For this review, take the finished solid that the model builds, in its own axes (mm). Face numbers are marked on the shaded views. A direction names the side the tool comes from. Round coordinates to 2 decimals unless told otherwise and drop trailing zeros. Write each loop counter-clockwise with the first axis right and the second up, starting at its lowest first coordinate (ties: lowest second). Pieces come first, ordered by that corner, then holes. Notation, with made-up numbers: (-22, 55.5) -> (26, 55.5) arc R14 cw to (26, 66.5) -> close; hole circle Ø4 at (38, 22). An arc over 180 degrees is marked (long way). Answer in a Markdown table with one row per item.
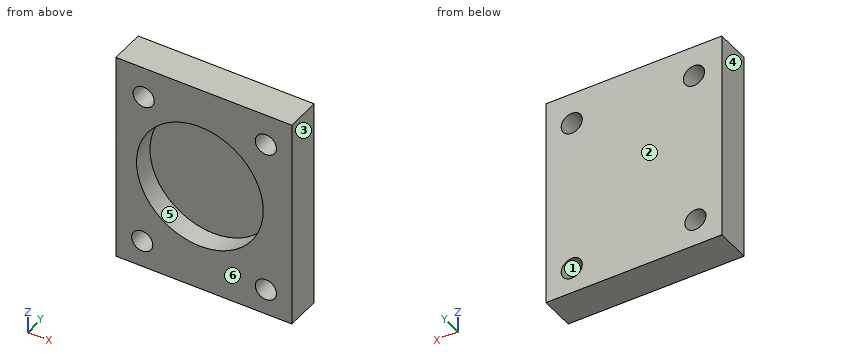
from build123d import *

# Parameters (mm, degrees)
F0_W     = 25
F0_H     = 30
F1_DEPTH = 5
F2_R     = 1.5
F3_DEPTH = 25
F4_R     = 9
F5_DEPTH = 3


with BuildPart() as f1:
    # F0 (on Front) → F1 (new body)
    with BuildSketch(Plane.XZ):
        with Locations((0.55913, 2.599103)):
            Rectangle(F0_W, F0_H)
    extrude(amount=F1_DEPTH)

    # F2 (on face) → F3 (cut)
    with BuildSketch(Plane.XZ.offset(5)):
        with Locations((-7.987171, 13.230707)):
            Circle(F2_R)
        with Locations((9.378917, 13.162337)):
            Circle(F2_R)
        with Locations((-8.192283, -8.579459)):
            Circle(F2_R)
        with Locations((9.378917, -8.716201)):
            Circle(F2_R)
    extrude(amount=-F3_DEPTH, mode=Mode.SUBTRACT)

    # F4 (on face) → F5 (cut)
    with BuildSketch(Plane.XZ.offset(5)):
        with Locations((0, 3.009328)):
            Circle(F4_R)
    extrude(amount=-F5_DEPTH, mode=Mode.SUBTRACT)


solid = f1.part
1) Consider section A-A on x = 0. State the section outline as (y, z) points.
Solved:
| item | result |
|---|---|
| outline | (-5, -12.4) -> (0, -12.4) -> (0, 17.6) -> (-5, 17.6) -> (-5, 12.01) -> (-2, 12.01) -> (-2, -5.99) -> (-5, -5.99) -> close |
2) Mouldability with a two-part tool opening along X and no side actions: class the marked faces 1, 2, 3 and 4 as pulls with the +X half, pulls with the -X half, needs draft (parallel to the pull), parting line crosses it, or undercut.
Solved:
| item | result |
|---|---|
| face 1 | undercut |
| face 2 | needs draft |
| face 3 | pulls with the +X half |
| face 4 | pulls with the -X half |
3) For the marked faces 5 and 6, list the 3-axis set-ups (+Z, -Z, +X, -X, +Y, -Y) from which the entire face can be reached by the end or side of a thin tool; tool diameter is ignored.
Solved:
| item | result |
|---|---|
| face 5 | -Y |
| face 6 | +Z, -Z, +X, -X, -Y |
4) For line 1 (Z direction, x = 8.25, y = -3.7); line 2 (Z direction, x = -7.5, y = -1.9); line 3 (X direction, y = -1.6, z = 12), list the stretches that pass through material, from the lowest coordinate up. Write a range as [from, to].
Solved:
| item | result |
|---|---|
| line 1 | [-12.4, -9.7], [-7.73, -0.59], [6.61, 12.17], [14.15, 17.6] |
| line 2 | [-12.4, -9.91], [-7.25, 11.81], [14.65, 17.6] |
| line 3 | [-11.94, -8.84], [-7.13, 8.43], [10.33, 13.06] |
5) Clearance check with flat-ended pins moving along their axes: pin 1 Ø4 at (x, z) = (9.38, -8.72) entering from -Y; pin 2 Ø5.5 at (x, z) = (-4.5, 1.5) entering from -Y. State where each tip first meets the part, or that it passes through.
Solved:
| item | result |
|---|---|
| pin 1 | y = -5 |
| pin 2 | y = -2 |
6) Consider section B-B on x = -7.75. State the section outline as (y, z) points, then the cut area to 3 significant figures.
Solved:
| item | result |
|---|---|
| outline | (-5, -12.4) -> (0, -12.4) -> (0, -10.01) -> (-5, -10.01) -> close; (-5, -7.15) -> (0, -7.15) -> (0, 11.75) -> (-5, 11.75) -> (-5, 7.59) -> (-2, 7.59) -> (-2, -1.57) -> (-5, -1.57) -> close; (-5, 14.71) -> (0, 14.71) -> (0, 17.6) -> (-5, 17.6) -> close |
| area | 93.4 mm² |
7) Consider section D-D on y = -0.9. State the section outline as (x, z) points, then the cut area to 3 significant figures.
Solved:
| item | result |
|---|---|
| outline | (-11.94, -12.4) -> (13.06, -12.4) -> (13.06, 17.6) -> (-11.94, 17.6) -> close; hole circle Ø3 at (-8.19, -8.58); hole circle Ø3 at (-7.99, 13.23); hole circle Ø3 at (9.38, -8.72); hole circle Ø3 at (9.38, 13.16) |
| area | 722 mm² |
8) Consider section C-C on y = -2.75. State the section outline as (x, z) points, then the cut area to 3 significant figures.
Solved:
| item | result |
|---|---|
| outline | (-11.94, -12.4) -> (13.06, -12.4) -> (13.06, 17.6) -> (-11.94, 17.6) -> close; hole circle Ø3 at (-8.19, -8.58); hole circle Ø3 at (-7.99, 13.23); hole circle Ø18 at (0, 3.01); hole circle Ø3 at (9.38, -8.72); hole circle Ø3 at (9.38, 13.16) |
| area | 467 mm² |
